Part model, mm, in its own coordinate system. A direction names the side the tool comes from. Round coordinates to 2 decimals unless told otherwise and drop trailing zeros. Write each loop counter-clockwise with the first axis right and the second up, starting at its lowest first coordinate (ties: lowest second). Pieces come first, ordered by that corner, then holes. Notation, with made-up numbers: (-21.75, 75) -> (5.25, 75) arc R4 cw to (5.25, 79) -> close; hole circle Ø4 at (53, 11.5). An arc over 180 degrees is marked (long way). Return JSON: item names as keys, results as strings. Group by question number.
(1) Drill centre lines: L1, parallel to Y at x = 31, z = 0; L2, parallel to X at y = -6.5, z = 8; L3, parallel to Y at x = 23, z = -3. Where is each one in solid material? Low to high. Write a range as from..to.
(2) Drop flat-ended pins along their axis: pin 1 Ø1.8 at (y, z) = (1.5, -0.5) entering from +X; pin 2 Ø1.5 at (x, z) = (36.5, -3.5) entering from -Y; pin 3 Ø8 at (x, y) = (33, 5.5) entering from +Z. Give the stop position or say it passes through.
(3) Saw through at B-B (y = 10.25). List the corners of the cut face in (x, z), plus the area to 3 significant figures.
(4) Mould opens along Z. For faces 4 (the cylindrical face through (2.112, 8.493, -1.886)), 5 (the cylindrical face through (21.101, -4.214, -0.553)), 6 (the flat face through (54, 0, 0)), 7 (the flat face through (58, -0.1, 3.3)) say: +Z half, -Z half, draft (parallel to the pull), parting line (faces both ways), or undercut.
(5) Tool access for faces 1 (the cylindrical face through (53.549, 8.493, -1.886)), 2 (the flat face through (10, -9, 2)), 3 (the cylindrical face through (30.3, -11.4, -1.5)): list every direction of +Z, -Z, +X, -X, +Y, -Y with a clear straight run to the whole face (end or side of a thin tool).
(6) Saw through at A-A (x = 35.5). List the corners of the cut face in (y, z).
from build123d import *

# Parameters (mm, degrees)
CUT_EXTRUDE_1_DEPTH = 4


with BuildPart() as part:
    # Эскиз3 → Повернуть1 (revolve)
    with BuildSketch(Plane.XY, mode=Mode.PRIVATE) as revolve_1_sk:
        Polygon((-7, 4.25), (-7, 7.7), (-6, 8.7), (10, 8.7), (10, 11.5), (50, 11.5), (50, 8.7), (57, 8.7), (58, 7.7), (58, 0), (52.453738644, 0), (50, 4.25), align=None)
    revolve(revolve_1_sk.sketch.rotate(Axis((-6.877569373, 0, 0), (1, 0, 0)), 90), axis=Axis((-6.877569373, 0, 0), (1, 0, 0)))

    # Эскиз4 → Вырез-Вытянуть1 (cut)
    with BuildSketch(Plane(origin=(58, 0, -31), x_dir=(0, 0, 1), z_dir=(-1, 0, 0))):
        with BuildLine():
            Line((30.778386531, 2.640717227), (30.875027145, 2.996524002))
            ThreePointArc((30.875027145, 2.996524002), (31, 2.999128925), (31.124972855, 2.996524002))
            Line((31.124972855, 2.996524002), (31.221613469, 2.640717227))
            ThreePointArc((31.221613469, 2.640717227), (31.345894409, 2.627328883), (31.469405738, 2.608094755))
            Line((31.469405738, 2.608094755), (31.654842973, 2.926765277))
            ThreePointArc((31.654842973, 2.926765277), (31.776231684, 2.896936085), (31.896271989, 2.862074568))
            Line((31.896271989, 2.862074568), (31.897530084, 2.493379183))
            ThreePointArc((31.897530084, 2.493379183), (32.014111096, 2.448280761), (32.12843572, 2.397734937))
            Line((32.12843572, 2.397734937), (32.390032334, 2.657552336))
            ThreePointArc((32.390032334, 2.657552336), (32.499564462, 2.597321838), (32.606491668, 2.532579481))
            Line((32.606491668, 2.532579481), (32.512281507, 2.176121468))
            ThreePointArc((32.512281507, 2.176121468), (32.613217787, 2.102386352), (32.710564672, 2.023973445))
            Line((32.710564672, 2.023973445), (33.030493289, 2.207231595))
            ThreePointArc((33.030493289, 2.207231595), (33.1207044, 2.1207044), (33.207231595, 2.030493289))
            Line((33.207231595, 2.030493289), (33.023973445, 1.710564672))
            ThreePointArc((33.023973445, 1.710564672), (33.102386352, 1.613217787), (33.176121468, 1.512281507))
            Line((33.176121468, 1.512281507), (33.532579481, 1.606491668))
            ThreePointArc((33.532579481, 1.606491668), (33.597321838, 1.499564462), (33.657552336, 1.390032334))
            Line((33.657552336, 1.390032334), (33.397734937, 1.12843572))
            ThreePointArc((33.397734937, 1.12843572), (33.448280761, 1.014111096), (33.493379183, 0.897530084))
            Line((33.493379183, 0.897530084), (33.862074568, 0.896271989))
            ThreePointArc((33.862074568, 0.896271989), (33.896936085, 0.776231684), (33.926765277, 0.654842973))
            Line((33.926765277, 0.654842973), (33.608094755, 0.469405738))
            ThreePointArc((33.608094755, 0.469405738), (33.627328883, 0.345894409), (33.640717227, 0.221613469))
            Line((33.640717227, 0.221613469), (33.996524002, 0.124972855))
            ThreePointArc((33.996524002, 0.124972855), (33.999128925, 0), (33.996524002, -0.124972855))
            Line((33.996524002, -0.124972855), (33.640717227, -0.221613469))
            ThreePointArc((33.640717227, -0.221613469), (33.627328883, -0.345894409), (33.608094755, -0.469405738))
            Line((33.608094755, -0.469405738), (33.926765277, -0.654842973))
            ThreePointArc((33.926765277, -0.654842973), (33.896936085, -0.776231684), (33.862074568, -0.896271989))
            Line((33.862074568, -0.896271989), (33.493379183, -0.897530084))
            ThreePointArc((33.493379183, -0.897530084), (33.448280761, -1.014111096), (33.397734937, -1.12843572))
            Line((33.397734937, -1.12843572), (33.657552336, -1.390032334))
            ThreePointArc((33.657552336, -1.390032334), (33.597321838, -1.499564462), (33.532579481, -1.606491668))
            Line((33.532579481, -1.606491668), (33.176121468, -1.512281507))
            ThreePointArc((33.176121468, -1.512281507), (33.102386352, -1.613217787), (33.023973445, -1.710564672))
            Line((33.023973445, -1.710564672), (33.207231595, -2.030493289))
            ThreePointArc((33.207231595, -2.030493289), (33.1207044, -2.1207044), (33.030493289, -2.207231595))
            Line((33.030493289, -2.207231595), (32.710564672, -2.023973445))
            ThreePointArc((32.710564672, -2.023973445), (32.613217787, -2.102386352), (32.512281507, -2.176121468))
            Line((32.512281507, -2.176121468), (32.606491668, -2.532579481))
            ThreePointArc((32.606491668, -2.532579481), (32.499564462, -2.597321838), (32.390032334, -2.657552336))
            Line((32.390032334, -2.657552336), (32.12843572, -2.397734937))
            ThreePointArc((32.12843572, -2.397734937), (32.014111096, -2.448280761), (31.897530084, -2.493379183))
            Line((31.897530084, -2.493379183), (31.896271989, -2.862074568))
            ThreePointArc((31.896271989, -2.862074568), (31.776231684, -2.896936085), (31.654842973, -2.926765277))
            Line((31.654842973, -2.926765277), (31.469405738, -2.608094755))
            ThreePointArc((31.469405738, -2.608094755), (31.345894409, -2.627328883), (31.221613469, -2.640717227))
            Line((31.221613469, -2.640717227), (31.124972855, -2.996524002))
            ThreePointArc((31.124972855, -2.996524002), (31, -2.999128925), (30.875027145, -2.996524002))
            Line((30.875027145, -2.996524002), (30.778386531, -2.640717227))
            ThreePointArc((30.778386531, -2.640717227), (30.654105591, -2.627328883), (30.530594262, -2.608094755))
            Line((30.530594262, -2.608094755), (30.345157027, -2.926765277))
            ThreePointArc((30.345157027, -2.926765277), (30.223768316, -2.896936085), (30.103728011, -2.862074568))
            Line((30.103728011, -2.862074568), (30.102469916, -2.493379183))
            ThreePointArc((30.102469916, -2.493379183), (29.985888904, -2.448280761), (29.87156428, -2.397734937))
            Line((29.87156428, -2.397734937), (29.609967666, -2.657552336))
            ThreePointArc((29.609967666, -2.657552336), (29.500435538, -2.597321838), (29.393508332, -2.532579481))
            Line((29.393508332, -2.532579481), (29.487718493, -2.176121468))
            ThreePointArc((29.487718493, -2.176121468), (29.386782213, -2.102386352), (29.289435328, -2.023973445))
            Line((29.289435328, -2.023973445), (28.969506711, -2.207231595))
            ThreePointArc((28.969506711, -2.207231595), (28.8792956, -2.1207044), (28.792768405, -2.030493289))
            Line((28.792768405, -2.030493289), (28.976026555, -1.710564672))
            ThreePointArc((28.976026555, -1.710564672), (28.897613648, -1.613217787), (28.823878532, -1.512281507))
            Line((28.823878532, -1.512281507), (28.467420519, -1.606491668))
            ThreePointArc((28.467420519, -1.606491668), (28.402678162, -1.499564462), (28.342447664, -1.390032334))
            Line((28.342447664, -1.390032334), (28.602265063, -1.12843572))
            ThreePointArc((28.602265063, -1.12843572), (28.551719239, -1.014111096), (28.506620817, -0.897530084))
            Line((28.506620817, -0.897530084), (28.137925432, -0.896271989))
            ThreePointArc((28.137925432, -0.896271989), (28.103063915, -0.776231684), (28.073234723, -0.654842973))
            Line((28.073234723, -0.654842973), (28.391905245, -0.469405738))
            ThreePointArc((28.391905245, -0.469405738), (28.372671117, -0.345894409), (28.359282773, -0.221613469))
            Line((28.359282773, -0.221613469), (28.003475998, -0.124972855))
            ThreePointArc((28.003475998, -0.124972855), (28.000871075, 0), (28.003475998, 0.124972855))
            Line((28.003475998, 0.124972855), (28.359282773, 0.221613469))
            ThreePointArc((28.359282773, 0.221613469), (28.372671117, 0.345894409), (28.391905245, 0.469405738))
            Line((28.391905245, 0.469405738), (28.073234723, 0.654842973))
            ThreePointArc((28.073234723, 0.654842973), (28.103063915, 0.776231684), (28.137925432, 0.896271989))
            Line((28.137925432, 0.896271989), (28.506620817, 0.897530084))
            ThreePointArc((28.506620817, 0.897530084), (28.551719239, 1.014111096), (28.602265063, 1.12843572))
            Line((28.602265063, 1.12843572), (28.342447664, 1.390032334))
            ThreePointArc((28.342447664, 1.390032334), (28.402678162, 1.499564462), (28.467420519, 1.606491668))
            Line((28.467420519, 1.606491668), (28.823878532, 1.512281507))
            ThreePointArc((28.823878532, 1.512281507), (28.897613648, 1.613217787), (28.976026555, 1.710564672))
            Line((28.976026555, 1.710564672), (28.792768405, 2.030493289))
            ThreePointArc((28.792768405, 2.030493289), (28.8792956, 2.1207044), (28.969506711, 2.207231595))
            Line((28.969506711, 2.207231595), (29.289435328, 2.023973445))
            ThreePointArc((29.289435328, 2.023973445), (29.386782213, 2.102386352), (29.487718493, 2.176121468))
            Line((29.487718493, 2.176121468), (29.393508332, 2.532579481))
            ThreePointArc((29.393508332, 2.532579481), (29.500435538, 2.597321838), (29.609967666, 2.657552336))
            Line((29.609967666, 2.657552336), (29.87156428, 2.397734937))
            ThreePointArc((29.87156428, 2.397734937), (29.985888904, 2.448280761), (30.102469916, 2.493379183))
            Line((30.102469916, 2.493379183), (30.103728011, 2.862074568))
            ThreePointArc((30.103728011, 2.862074568), (30.223768316, 2.896936085), (30.345157027, 2.926765277))
            Line((30.345157027, 2.926765277), (30.530594262, 2.608094755))
            ThreePointArc((30.530594262, 2.608094755), (30.654105591, 2.627328883), (30.778386531, 2.640717227))
        make_face()
    extrude(amount=CUT_EXTRUDE_1_DEPTH, mode=Mode.SUBTRACT)


solid = part.part
Computed values:
{
 "1": {"L1": "-11.5..-4.25, 4.25..11.5", "L2": "10..50", "L3": "-11.1..-3.01, 3.01..11.1"},
 "2": {"pin 1": "x = 54", "pin 2": "y = -11.17", "pin 3": "z = 11.4"},
 "3": {"outline": "(10, -5.21) -> (50, -5.21) -> (50, 5.21) -> (10, 5.21) -> close", "area": "417 mm2"},
 "4": {"face 4": "parting line", "face 5": "undercut", "face 6": "undercut", "face 7": "draft"},
 "5": {"face 1": "+X", "face 2": "-X", "face 3": "+X, -X"},
 "6": {"outline": "circle Ø23 at (0, 0); hole circle Ø8.5 at (0, 0)"}
}
